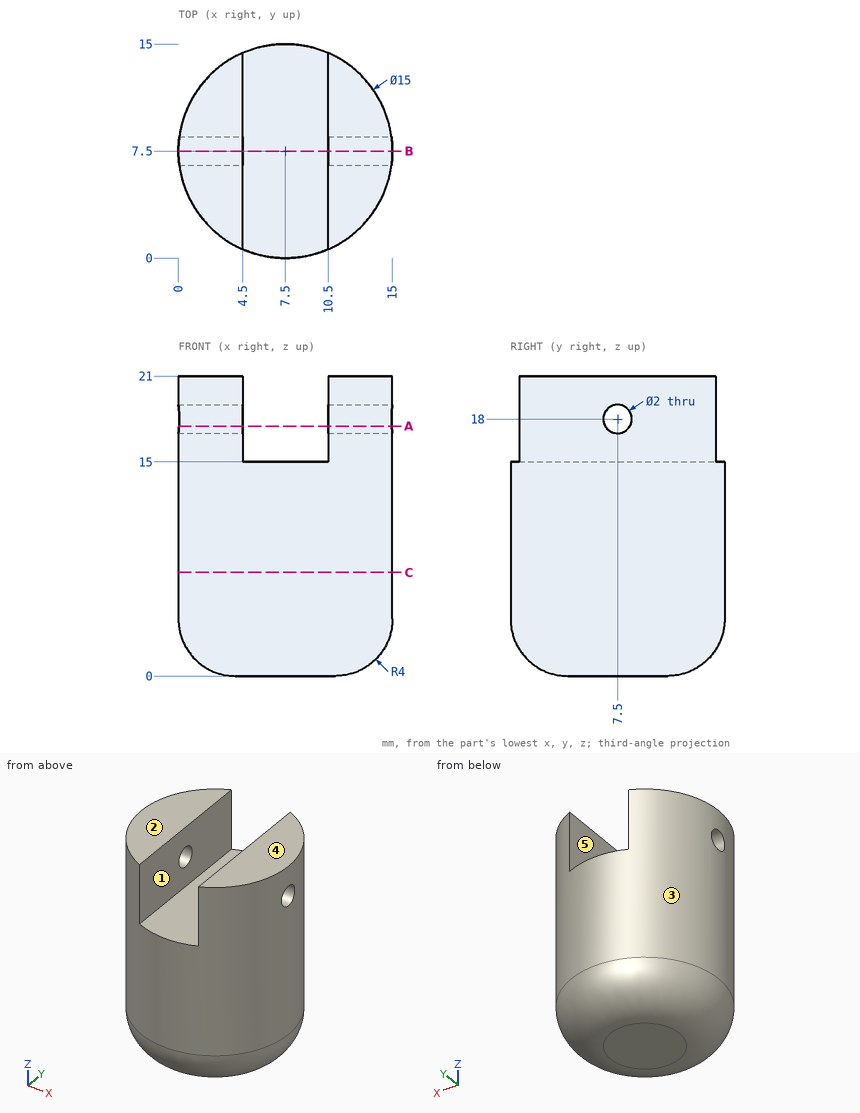
Job drawing, mm, ordinate dimensions from the low corner. One solid piece. A direction names the side the tool comes from. Give positions to 0.01 mm unless a question says otherwise; leave off trailing zeros. Write each loop counter-clockwise with the first axis right and the second up, starting at its lowest first coordinate (ties: lowest second). Pieces come first, ordered by that corner, then holes. Notation, with made-up numbers: M -9.5,-23 L -2.5,-23 A28 ccw -2.5,13 Z; hole C -18.75,5.5 d1. An arc over 180 degrees is marked long. One line per item, written item: value. Start each with the question number.
Q1. 3-axis set-ups, long thin cutter, end or side, ignore diameter. For the marked faces 1 and 2: which of +Z, -Z, +X, -X, +Y, -Y reach the whole face in a straight line?
Q2. Saw through at A-A, the plane z = 17.5. Write the cut outline in (x, y), plus the area to 3 significant figures.
Q3. Saw through at B-B, the plane y = 7.5. State how many separate pieces and enclosed holes the cut face has, plus the area to 3 significant figures.
Q4. Two-plate mould, pull along X, no slides. Class the marked faces 3, 4 and 5: +X half, -X half, draft (parallel to the pull), parting line (faces both ways), or undercut.
Q5. Probe probe 1 along X at (y, z) = (4.25, 17); probe 2 along X at (y, z) = (3.25, 18.5); probe 3 along Z at (x, y) = (4, 8). List the from-to ranges inside material, lowest first. Write a range as [from, to].
Q6. Drop flat-ended pins along their axis: pin 1 Ø2 at (y, z) = (4, 10.5) entering from -X; pin 2 Ø1 at (y, z) = (5.5, 5) entering from +X; pin 3 Ø2 at (x, y) = (3.5, 11.5) entering from -Z; pin 4 Ø1.6 at (y, z) = (7.5, 18) entering from +X. Give the stop position or say it passes through.
Q7. Saw through at C-C, the plane z = 7.25. Write the cut outline in (x, y).
Output values:
1. face 1: +Z, +Y, -Y
1. face 2: +Z, +X, -X, +Y, -Y
2. outline: M 0.05,6.63 A7.5 ccw 4.5,0.63 L 4.5,6.63 Z; M 0.05,8.37 L 4.5,8.37 L 4.5,14.37 A7.5 ccw Z; M 10.5,0.63 A7.5 ccw 14.95,6.63 L 10.5,6.63 Z; M 10.5,8.37 L 14.95,8.37 A7.5 ccw 10.5,14.37 Z
2. area: 73.6 mm²
3. separate pieces: 3
3. enclosed holes: 0
3. area: 254 mm²
4. face 3: parting line
4. face 4: draft
4. face 5: undercut
5. probe 1: x = [0.74, 4.5], [10.5, 14.26]
5. probe 2: x = [1.32, 4.5], [10.5, 13.68]
5. probe 3: z = [0, 17.13], [18.87, 21]
6. pin 1: stops at x = 0.43
6. pin 2: stops at x = 14.85
6. pin 3: stops at z = 0.17
6. pin 4: passes through
7. outline: C 7.5,7.5 d15
